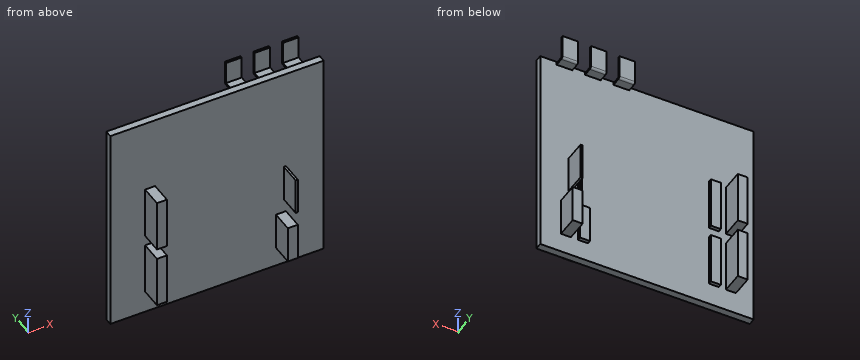
```python
from build123d import *

# Parameters (mm, degrees)
SKETCH1_W           = 76.2
SKETCH1_H           = 76.2
EXTRUDE1_DEPTH      = 2.54
SKETCH2_W           = 3.556
SKETCH2_H           = 13.462
SKETCH2_W_2         = 0.762
SKETCH2_H_2         = 13.208
SKETCH2_H_3         = 18.796
EXTRUDE2_DEPTH      = 1.27
EXTRUDE2_DEPTH_BACK = 10.1601
SKETCH3_W           = 5.588
SKETCH3_H           = 0.762
EXTRUDE3_DEPTH      = 3.048
LPATTERN1_COUNT     = 3
LPATTERN1_PITCH     = 10.16
SKETCH8_W           = 5.588
SKETCH8_H           = 0.762
REVOLVE3_ANGLE      = 90
SKETCH9_W           = 5.588
SKETCH9_H           = 0.762
EXTRUDE5_DEPTH      = 8.128
LPATTERN2_COUNT     = 3
LPATTERN2_PITCH     = 10.16
SKETCH11_W          = 3.556
SKETCH11_H          = 18.796
SKETCH11_W_2        = 0.762
SKETCH11_H_2        = 13.208
SKETCH11_H_3        = 13.462
EXTRUDE6_DEPTH      = 6.35
SKETCH12_W          = 3.556
SKETCH12_H          = 18.796
SKETCH12_H_2        = 13.462
SKETCH12_W_2        = 0.762
SKETCH12_H_3        = 13.208
EXTRUDE7_DEPTH      = 7.6201


with BuildPart() as part:
    # Sketch1 → Extrude1 (new body)
    with BuildSketch(Plane(origin=(0, 0, 0), x_dir=(1, 0, 0), z_dir=(0, 1, 0))):
        Rectangle(SKETCH1_W, SKETCH1_H)
    extrude(amount=EXTRUDE1_DEPTH)

    # Sketch2 → Extrude2 (add, two sides)
    with BuildSketch(Plane(origin=(0, 2.54, 0), x_dir=(-1, 0, 0), z_dir=(0, 1, 0))) as extrude2_sk:
        with Locations((-22.86, -24.257)):
            Rectangle(SKETCH2_W, SKETCH2_H)
        with Locations((-24.257, -5.842)):
            Rectangle(SKETCH2_W_2, SKETCH2_H_2)
        with Locations((23.876, -20.574)):
            Rectangle(SKETCH2_W, SKETCH2_H_3)
        with Locations((23.876, 2.032)):
            Rectangle(SKETCH2_W, SKETCH2_H_3)
        with Locations((29.972, -20.574)):
            Rectangle(SKETCH2_W, SKETCH2_H_3)
        with Locations((29.972, 2.032)):
            Rectangle(SKETCH2_W, SKETCH2_H_3)
        with Locations((-28.956, -24.257)):
            Rectangle(SKETCH2_W, SKETCH2_H)
        with Locations((-27.559, -5.842)):
            Rectangle(SKETCH2_W_2, SKETCH2_H_2)
    extrude(amount=EXTRUDE2_DEPTH)
    extrude(extrude2_sk.sketch, amount=-EXTRUDE2_DEPTH_BACK)

    # Sketch3 → Extrude3 (add)
    with BuildSketch(Plane(origin=(0, 2.54, 0), x_dir=(-1, 0, 0), z_dir=(0, 1, 0))):
        with Locations((-9.144, 37.338)):
            Rectangle(SKETCH3_W, SKETCH3_H)
    extrude3 = extrude(amount=EXTRUDE3_DEPTH)

    # LPattern1: Extrude3 ×3
    with Locations(*[(i * LPATTERN1_PITCH, 0, 0) for i in range(1, LPATTERN1_COUNT)]):
        add(extrude3)

    # Sketch8 → Revolve3 (revolve)
    with BuildSketch(Plane(origin=(0, 5.588, 0), x_dir=(1, 0, 0), z_dir=(0, 1, 0))):
        with Locations((9.144, -37.338)):
            Rectangle(SKETCH8_W, SKETCH8_H)
        with Locations((19.304, -37.338)):
            Rectangle(SKETCH8_W, SKETCH8_H)
        with Locations((29.464, -37.338)):
            Rectangle(SKETCH8_W, SKETCH8_H)
    revolve(axis=Axis((6.35, 5.588, 37.719), (1, 0, 0)), revolution_arc=REVOLVE3_ANGLE)

    # Sketch9 → Extrude5 (add)
    with BuildSketch(Plane.XY.offset(37.719)):
        with Locations((9.144, 5.969)):
            Rectangle(SKETCH9_W, SKETCH9_H)
    extrude5 = extrude(amount=EXTRUDE5_DEPTH)

    # LPattern2: Extrude5 ×3
    with Locations(*[(i * LPATTERN2_PITCH, 0, 0) for i in range(1, LPATTERN2_COUNT)]):
        add(extrude5)

    # Sketch11 → Extrude6 (add)
    with BuildSketch(Plane(origin=(0, 3.81, 0), x_dir=(1, 0, 0), z_dir=(0, 1, 0))):
        with Locations((-29.972, 20.574)):
            Rectangle(SKETCH11_W, SKETCH11_H)
        with Locations((-29.972, -2.032)):
            Rectangle(SKETCH11_W, SKETCH11_H)
        with Locations((27.559, 5.842)):
            Rectangle(SKETCH11_W_2, SKETCH11_H_2)
        with Locations((28.956, 24.257)):
            Rectangle(SKETCH11_W, SKETCH11_H_3)
    extrude(amount=EXTRUDE6_DEPTH)

    # Sketch12 → Extrude7 (cut)
    with BuildSketch(Plane.XZ.offset(7.6201)):
        with Locations((-29.972, -20.574)):
            Rectangle(SKETCH12_W, SKETCH12_H)
        with Locations((-29.972, 2.032)):
            Rectangle(SKETCH12_W, SKETCH12_H)
        with Locations((28.956, -24.257)):
            Rectangle(SKETCH12_W, SKETCH12_H_2)
        with Locations((27.559, -5.842)):
            Rectangle(SKETCH12_W_2, SKETCH12_H_3)
    extrude(amount=-EXTRUDE7_DEPTH, mode=Mode.SUBTRACT)


solid = part.part
```
Geometry: final body of the model. Coordinates: model frame, mm. Coordinates: 2 decimals unless noted, no trailing zeros. Order: outer loops, then holes, each group sorted by start corner. A loop starts at its lowest first (then second) coordinate and runs counter-clockwise, first axis right, second up. Notation, with made-up numbers: (80.5, 16) - (84.5, 16) arc R23 ccw to (84.5, 24) - close; hole circle Ø7 at (-3.5, 42.25). An arc over 180 degrees is marked (long way). Return JSON: item names as keys, results as strings. Group by question number.
1. Cut plane B-B (z = -20.5). Output: boundary loops of the cut face in (x, y).
2. Pin query (flat end, axial travel): pin 1 (0.6 mm diameter, centred on x = -23.5, y = 3, fed in from +Z); pin 2 (1.1 mm diameter, centred on x = -23, y = -4.5, fed in from -Z); pin 3 (6 mm diameter, centred on y = 7, z = 5, fed in from -X). Return the tip coordinate at first contact, or that it passes through.
3. Cut plane A-A (y = -1.75). Output: boundary loops of the cut face in (x, z), plus the area to 3 significant figures.
4. Material intervals for line 1 along X through (y, z) = (-5.75, -28.5); line 2 along Z through (x, y) = (-14, 2.25); line 3 along X through (y, z) = (-4, -14.5), sorted ascending. Write a range as [from, to].
5. Cut plane D-D (z = -2). Output: boundary loops of the cut face in (x, y).
6. Cut plane C-C (x = -33). Output: boundary loops of the cut face in (y, z), plus the area to 3 significant figures.
Resolved:
{
 "1": {"outline": "(-38.1, 0) - (-25.65, 0) - (-25.65, -7.62) - (-22.1, -7.62) - (-22.1, 0) - (21.08, 0) - (21.08, -7.62) - (24.64, -7.62) - (24.64, 0) - (38.1, 0) - (38.1, 2.54) - (30.73, 2.54) - (30.73, 10.16) - (27.18, 10.16) - (27.18, 2.54) - (24.64, 2.54) - (24.64, 3.81) - (21.08, 3.81) - (21.08, 2.54) - (-22.1, 2.54) - (-22.1, 3.81) - (-25.65, 3.81) - (-25.65, 2.54) - (-28.19, 2.54) - (-28.19, 10.16) - (-31.75, 10.16) - (-31.75, 2.54) - (-38.1, 2.54) - close"},
 "2": {"pin 1": "stops at z = 11.43", "pin 2": "stops at z = -29.97", "pin 3": "stops at x = -31.75"},
 "3": {"outline": "(-25.65, -29.97) - (-22.1, -29.97) - (-22.1, -11.18) - (-25.65, -11.18) - close; (-25.65, -7.37) - (-22.1, -7.37) - (-22.1, 11.43) - (-25.65, 11.43) - close; (21.08, -30.99) - (24.64, -30.99) - (24.64, -17.53) - (21.08, -17.53) - close; (23.88, -12.45) - (24.64, -12.45) - (24.64, 0.76) - (23.88, 0.76) - close", "area": "192 mm²"},
 "4": {"line 1": "x = [-25.65, -22.1], [21.08, 24.64]", "line 2": "z = [-38.1, 38.1]", "line 3": "x = [-25.65, -22.1]"},
 "5": {"outline": "(-38.1, 0) - (-25.65, 0) - (-25.65, -7.62) - (-22.1, -7.62) - (-22.1, 0) - (23.88, 0) - (23.88, -7.62) - (24.64, -7.62) - (24.64, 0) - (38.1, 0) - (38.1, 2.54) - (27.94, 2.54) - (27.94, 10.16) - (27.18, 10.16) - (27.18, 2.54) - (24.64, 2.54) - (24.64, 3.81) - (23.88, 3.81) - (23.88, 2.54) - (-22.1, 2.54) - (-22.1, 3.81) - (-25.65, 3.81) - (-25.65, 2.54) - (-28.19, 2.54) - (-28.19, 10.16) - (-31.75, 10.16) - (-31.75, 2.54) - (-38.1, 2.54) - close"},
 "6": {"outline": "(0, -38.1) - (2.54, -38.1) - (2.54, 38.1) - (0, 38.1) - close", "area": "194 mm²"}
}
